Read the model definition and answer for the solid it produces. Units are mm, in the model's axes. A direction names the side the tool comes from. Coordinates: 2 decimals unless noted, no trailing zeros. Write each loop counter-clockwise with the first axis right and the second up, starting at its lowest first coordinate (ties: lowest second). Pieces come first, ordered by that corner, then holes. Notation, with made-up numbers: (-24, 7.5) -> (-19, 7.5) arc R24 cw to (-19, 23.5) -> close; hole circle Ø11 at (-38, 16.25). An arc over 180 degrees is marked (long way). Return JSON: item names as keys, results as strings.
from build123d import *

# Parameters (mm, degrees)
EXTRUDE_1_DEPTH = 18


with BuildPart() as part:
    # 草图1 → 凸台-拉伸1 (new body)
    with BuildSketch(Plane.XY):
        with BuildLine():
            Line((-70, -67.5), (-8.660254038, -67.5))
            Line((-8.660254038, -67.5), (-8.660254038, -62.5))
            Line((-8.660254038, -62.5), (8.660254038, -62.5))
            Line((8.660254038, -62.5), (8.660254038, -67.5))
            Line((8.660254038, -67.5), (70, -67.5))
            ThreePointArc((70, -67.5), (73.535533906, -66.035533906), (75, -62.5))
            Line((75, -62.5), (75, 62.5))
            ThreePointArc((75, 62.5), (73.535533906, 66.035533906), (70, 67.5))
            Line((70, 67.5), (-70, 67.5))
            ThreePointArc((-70, 67.5), (-73.535533906, 66.035533906), (-75, 62.5))
            Line((-75, 62.5), (-75, -62.5))
            ThreePointArc((-75, -62.5), (-73.535533906, -66.035533906), (-70, -67.5))
        make_face()
    extrude(amount=EXTRUDE_1_DEPTH)


solid = part.part
1. A flat-ended cylindrical pin translates along its axis: pin 1 Ø4 at (y, z) = (-65, 11) entering from +X. Find the tip coordinate at first contact, or state that the pin passes through.
Taken from the geometry:
{"pin 1": "stops at x = 74.97"}
2. For a pull along X with two mould halves and no side action, classify faces 3 (the face through (-75, 1, 9)), 4 (the face through (-8.66, -65, 9)), 5 (the face through (-1, 1, 0)) as +X half, -X half, draft (parallel to the pull), parting line (faces both ways), or undercut.
Taken from the geometry:
{"face 3": "-X half", "face 4": "undercut", "face 5": "draft"}
3. A tool of negligible diameter and unlimited length cuts with its end or side. For faces 1 (the face through (39, -67.5, 9)), 2 (the face through (0, -62.5, 9)), from which of +Z, -Z, +X, -X, +Y, -Y can it reach the whole face along a straight path? Write none if from no direction.
Taken from the geometry:
{"face 1": "+Z, -Z, +X, -X, -Y", "face 2": "+Z, -Z, -Y"}
4. The part is cut by section A-A (x = 1.5). Determine the outline of the cut face in (y, z), then the cut area to 3 significant figures.
Taken from the geometry:
{"outline": "(-62.5, 0) -> (67.5, 0) -> (67.5, 18) -> (-62.5, 18) -> close", "area": "2,340 mm2"}
5. Consider L1, parallel to Y at x = 2.5, z = 16.75. Determine where the line is inside the solid, lowest interval first.
Taken from the geometry:
{"L1": "y = -62.5 to 67.5"}
